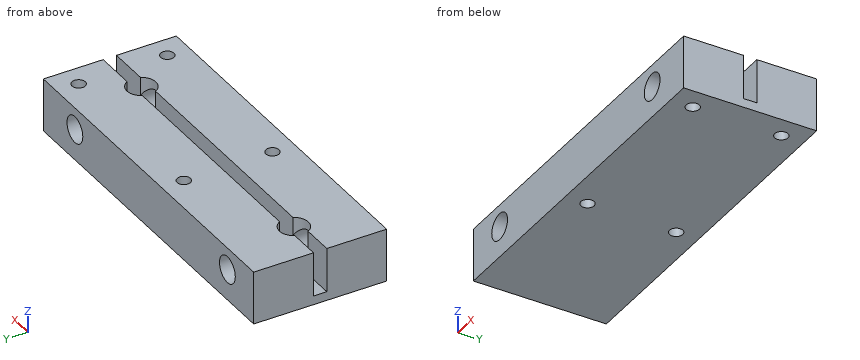
```python
from build123d import *

# Parameters (mm, degrees)
F0_W     = 80
F0_H     = 30
F1_DEPTH = 12
F2_R     = 1.5
F3_DEPTH = 25
F5_DEPTH = 5
F6_DEPTH = 10
F7_R     = 3
F8_DEPTH = 30.001


with BuildPart() as f1:
    # F0 (on Top) → F1 (new body)
    with BuildSketch(Plane.XY):
        with Locations((40, 15)):
            Rectangle(F0_W, F0_H)
    extrude(amount=F1_DEPTH)

    # F2 (on face) → F3 (cut)
    with BuildSketch(Plane.XY.offset(12)):
        with Locations((35, 5)):
            Circle(F2_R)
        with Locations((35, 25)):
            Circle(F2_R)
        with Locations((75, 5)):
            Circle(F2_R)
        with Locations((75, 25)):
            Circle(F2_R)
    extrude(amount=-F3_DEPTH, mode=Mode.SUBTRACT)

    # F4 (on face) → F5 (cut)
    with BuildSketch(Plane.XY.offset(12)):
        with BuildLine():
            Line((42.8169872981, 13.5), (65.1168593513, 13.5))
            ThreePointArc((65.1168593513, 13.5), (68, 11.75), (70.8831406487, 13.5))
            Line((70.8831406487, 13.5), (80, 13.5))
            Line((80, 13.5), (80, 16.5))
            Line((80, 16.5), (70.8831406487, 16.5))
            ThreePointArc((70.8831406487, 16.5), (68, 18.25), (65.1168593513, 16.5))
            Line((65.1168593513, 16.5), (42.8169872981, 16.5))
            Line((42.8169872981, 16.5), (12.8831406487, 16.5))
            ThreePointArc((12.8831406487, 16.5), (10, 18.25), (7.1168593513, 16.5))
            Line((7.1168593513, 16.5), (0, 16.5))
            Line((0, 16.5), (0, 13.5))
            Line((0, 13.5), (7.1168593513, 13.5))
            ThreePointArc((7.1168593513, 13.5), (10, 11.75), (12.8831406487, 13.5))
            Line((12.8831406487, 13.5), (42.8169872981, 13.5))
        make_face()
    extrude(amount=-F5_DEPTH, mode=Mode.SUBTRACT)

    # F4 (on face) → F6 (cut)
    with BuildSketch(Plane.XY.offset(12)):
        with BuildLine():
            Line((42.8169872981, 13.5), (65.1168593513, 13.5))
            ThreePointArc((65.1168593513, 13.5), (68, 11.75), (70.8831406487, 13.5))
            Line((70.8831406487, 13.5), (80, 13.5))
            Line((80, 13.5), (80, 16.5))
            Line((80, 16.5), (70.8831406487, 16.5))
            ThreePointArc((70.8831406487, 16.5), (68, 18.25), (65.1168593513, 16.5))
            Line((65.1168593513, 16.5), (42.8169872981, 16.5))
            Line((42.8169872981, 16.5), (12.8831406487, 16.5))
            ThreePointArc((12.8831406487, 16.5), (10, 18.25), (7.1168593513, 16.5))
            Line((7.1168593513, 16.5), (0, 16.5))
            Line((0, 16.5), (0, 13.5))
            Line((0, 13.5), (7.1168593513, 13.5))
            ThreePointArc((7.1168593513, 13.5), (10, 11.75), (12.8831406487, 13.5))
            Line((12.8831406487, 13.5), (42.8169872981, 13.5))
        make_face()
    extrude(amount=-F6_DEPTH, mode=Mode.SUBTRACT)

    # F7 (on face) → F8 (cut, through all)
    with BuildSketch(Plane(origin=(0, 30, 0), x_dir=(-1, 0, 0), z_dir=(0, 1, 0))):
        with Locations((-68, 7)):
            Circle(F7_R)
        with Locations((-10, 7)):
            Circle(F7_R)
    extrude(amount=-F8_DEPTH, mode=Mode.SUBTRACT)


solid = f1.part
```
Work out the finished part from the listing and answer in its coordinate system (mm). Coordinates: 2 decimals unless noted, no trailing zeros. Loops run counter-clockwise (first coordinate to the right, second up) from the corner with the lowest first, then second, coordinate; pieces in that order, holes last. Notation, with made-up numbers: M 55.25,-25.75 L 90.25,-25.75 A8 cw 90.25,-10.75 Z; hole C 40.25,51 d10. An arc over 180 degrees is marked long. Use CSV: the item, a comma, the result in double quotes. Start each with the question number.
(1) Find section A-A, the plane z = 7. State how many separate pieces and enclosed holes the cut face has, then the cut area to 3 significant figures.
(2) Find section B-B, the plane y = 5. Give the vertices of the cut face in (x, z), then the cut area to 3 significant figures.
(3) Find section D-D, the plane x = 42.5. Give the vertices of the cut face in (y, z).
(4) Find section C-C, the plane x = 68. Give the vertices of the cut face in (y, z), then the cut area to 3 significant figures.
(5) Given pin 1 Ø3.5 at (x, y) = (75, 5) entering from +Z; pin 2 Ø3.5 at (x, z) = (68, 7) entering from +Y, each flat-ended and moving along its own axis, determine where each tip first touches the part or whether it passes through.
(6) Consider line 1 (Y direction, x = 35, z = 3.5); line 2 (Y direction, x = 26, z = 7.75); line 3 (X direction, y = 23, z = 7). Determine where each line is inside the solid, lowest interval first.
Recorded:
1,separate pieces,"6"
1,enclosed holes,"4"
1,area,"1,810 mm^2"
2,outline,"M 0,0 L 33.5,0 L 33.5,12 L 0,12 Z; M 36.5,0 L 73.5,0 L 73.5,12 L 36.5,12 Z; M 76.5,0 L 80,0 L 80,12 L 76.5,12 Z; hole C 10,7 d6; hole C 68,7 d6"
2,area,"831 mm^2"
3,outline,"M 0,0 L 30,0 L 30,12 L 16.5,12 L 16.5,2 L 13.5,2 L 13.5,12 L 0,12 Z"
4,outline,"M 0,0 L 30,0 L 30,4 L 18.25,4 L 18.25,2 L 11.75,2 L 11.75,4 L 0,4 Z; M 0,10 L 11.75,10 L 11.75,12 L 0,12 Z; M 18.25,10 L 30,10 L 30,12 L 18.25,12 Z"
4,area,"154 mm^2"
5,pin 1,"stops at z = 12"
5,pin 2,"passes through"
6,line 1,"y = 0 to 3.5, 6.5 to 13.5, 16.5 to 23.5, 26.5 to 30"
6,line 2,"y = 0 to 13.5, 16.5 to 30"
6,line 3,"x = 0 to 7, 13 to 65, 71 to 80"
